```python
from build123d import *

# Parameters (mm, degrees)
HEAD_EXTRUDE_DEPTH        = 3.175
HEAD_EXTRUDE_DEPTH_BACK   = 3.175
HANDLE_EXTRUDE_DEPTH      = 2.2225
HANDLE_EXTRUDE_DEPTH_BACK = 2.2225


with BuildPart() as part:
    # head _ handle sketch → head extrude (new, two sides: drawn at the far end of the back side and taken through both)
    with BuildSketch(Plane(origin=(0, 0, 0), x_dir=(0, 1, 0), z_dir=(0, 0, 1)).offset(-HEAD_EXTRUDE_DEPTH_BACK)):
        with BuildLine():
            ThreePointArc((1.854333587, -17.097601941), (-6.685826637, -15.212601851), (-14.08039185, -10.542701714))
            Line((-14.08039185, -10.542701714), (1.37833241, -7.81691154))
            ThreePointArc((1.37833241, -7.81691154), (4.236175861, 0.746952099), (-1.37833241, 7.81691154))
            Line((-1.37833241, 7.81691154), (-16.837056671, 5.091121365))
            ThreePointArc((-16.837056671, 5.091121365), (-11.48563822, 12.008482318), (-4.105220678, 16.700709816))
            ThreePointArc((-4.105220678, 16.700709816), (4.627386809, 17.067655437), (11.52906135, 11.704823057))
            ThreePointArc((11.52906135, 11.704823057), (15.008470156, 2.646398228), (14.837059135, -7.055764638))
            ThreePointArc((14.837059135, -7.055764638), (10.185803197, -14.455690369), (1.854333587, -17.097601941))
        make_face()
    extrude(amount=HEAD_EXTRUDE_DEPTH + HEAD_EXTRUDE_DEPTH_BACK)

    # Sketch2_3 → handle extrude (add, two sides: drawn at the far end of the back side and taken through both)
    with BuildSketch(Plane(origin=(0, 0, 0), x_dir=(0, 1, 0), z_dir=(0, 0, 1)).offset(-HANDLE_EXTRUDE_DEPTH_BACK)):
        with BuildLine():
            ThreePointArc((49.692005566, 6.6675), (27.402174057, 9.142712932), (6.198407098, 16.44774781))
            ThreePointArc((6.198407098, 16.44774781), (9.203666438, 14.458341062), (11.52906135, 11.704823057))
            ThreePointArc((11.52906135, 11.704823057), (15.008470156, 2.646398228), (14.837059135, -7.055764638))
            ThreePointArc((14.837059135, -7.055764638), (12.331168475, -12.345606251), (7.718992867, -15.94973561))
            ThreePointArc((7.718992867, -15.94973561), (28.430370524, -9.015182994), (50.145286343, -6.6675))
            Line((50.145286343, -6.6675), (145.898407098, -6.6675))
            ThreePointArc((145.898407098, -6.6675), (155.798350359, -8.042920845), (164.948407098, -12.065))
            Line((164.948407098, -12.065), (164.948407098, 12.065))
            ThreePointArc((164.948407098, 12.065), (155.798350359, 8.042920845), (145.898407098, 6.6675))
            Line((145.898407098, 6.6675), (49.692005566, 6.6675))
        make_face()
    extrude(amount=HANDLE_EXTRUDE_DEPTH + HANDLE_EXTRUDE_DEPTH_BACK)


solid = part.part
```
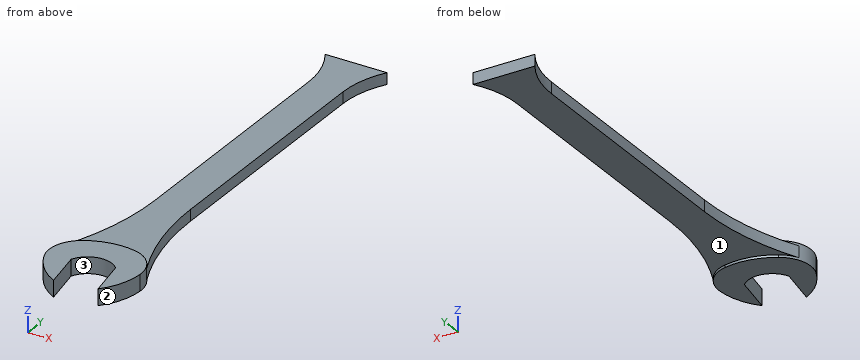
For this review, take the finished solid that the model builds, in its own axes (mm). Face numbers are marked on the shaded views. Coordinates: 2 decimals unless noted, no trailing zeros. Order: outer loops, then holes, each group sorted by start corner. A loop starts at its lowest first (then second) coordinate and runs counter-clockwise, first axis right, second up. Notation, with made-up numbers: (20.25, -14) -> (46.25, -14) arc R25 cw to (46.25, 7) -> close; hole circle Ø9 at (41.5, 60). An arc over 180 degrees is marked (long way). Use CSV: the item, a comma, the result in double quotes. Start each with the question number.
Item 1: We need section A-A, the plane z = 0. Give the boundary of the cut face in (x, y) (1 decimal), then the cut area to 3 significant figures.
Item 2: Wall thickness on probe 1 along Z at (x, y) = (-3, 32.5); probe 2 along X at (y, z) = (135, 0.75); probe 3 along Y at (x, z) = (1, 1.25): over which ranges is each line inside the solid? List them lowest first.
Item 3: We need section D-D, the plane y = 106. Give the boundary of the cut face in (x, z).
Item 4: We need section B-B, the plane x = -9.5. Give the boundary of the cut face in (y, z) (1 decimal), then the cut area to 3 significant figures.
Item 5: Insertion check: pin 1 (1 mm diameter, centred on y = 136.5, z = 0.5, fed in from -X); pin 2 (8 mm diameter, centred on x = 5.5, y = 106, fed in from +Z); pin 3 (3 mm diameter, centred on y = 104, z = -2, fed in from +X). Each pin has a flat end and moves straight along its axis. Give the tip position at first contact, or say it passes through.
Item 6: We need section C-C, the plane x = 3.5. Give the boundary of the cut face in (y, z) (1 decimal).
Item 7: Draft analysis for pull direction Y (two halves, no side actions). For the marked faces 1, 2 and 3, state which applies: pulls with the +Y half, pulls with the -Y half, needs draft (parallel to the pull), parting line crosses it, or undercut.
Derived:
1,outline,"(-16.7, -4.1) arc R25.4 ccw to (-5.1, -16.8) -> (-7.8, -1.4) arc R9.5 cw to (7.8, 1.4) -> (10.5, -14.1) arc R25.4 ccw to (17.1, 1.9) arc R12.7 ccw to (15.9, 7.7) arc R101.6 cw to (6.7, 50.1) -> (6.7, 145.9) arc R36.3 cw to (12.1, 164.9) -> (-12.1, 164.9) arc R36.3 cw to (-6.7, 145.9) -> (-6.7, 49.7) arc R101.6 cw to (-16.4, 6.2) arc R12.7 ccw to start"
1,area,"2,820 mm^2"
2,probe 1,"z = -2.22 to 2.22"
2,probe 2,"x = -6.67 to 6.67"
2,probe 3,"y = 4.38 to 164.95"
3,outline,"(-6.67, -2.22) -> (6.67, -2.22) -> (6.67, 2.22) -> (-6.67, 2.22) -> close"
4,outline,"(-13.9, -3.2) -> (12.8, -3.2) -> (12.8, -2.2) -> (25.9, -2.2) -> (25.9, 2.2) -> (12.8, 2.2) -> (12.8, 3.2) -> (-13.9, 3.2) -> close; (160, -2.2) -> (164.9, -2.2) -> (164.9, 2.2) -> (160, 2.2) -> close"
4,area,"250 mm^2"
5,pin 1,"stops at x = -6.67"
5,pin 2,"stops at z = 2.22"
5,pin 3,"stops at x = 6.67"
6,outline,"(4, -3.2) -> (15.3, -3.2) -> (15.3, -2.2) -> (164.9, -2.2) -> (164.9, 2.2) -> (15.3, 2.2) -> (15.3, 3.2) -> (4, 3.2) -> close"
7,face 1,"needs draft"
7,face 2,"pulls with the -Y half"
7,face 3,"undercut"
